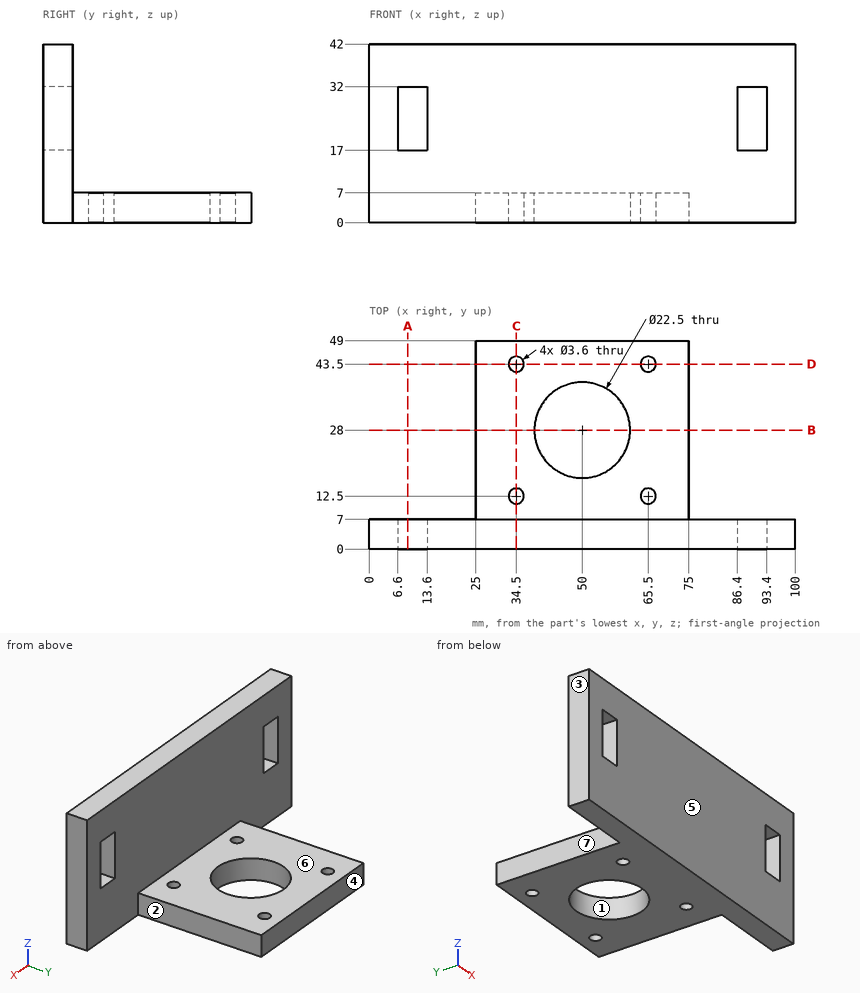
Job drawing, mm, ordinate dimensions from the low corner. One solid piece. A direction names the side the tool comes from. Give positions to 0.01 mm unless a question says otherwise; leave off trailing zeros. Order: outer loops, then holes, each group sorted by start corner. A loop starts at its lowest first (then second) coordinate and runs counter-clockwise, first axis right, second up. Notation, with made-up numbers: (15.5, 88.5) -> (38.5, 88.5) arc R23 ccw to (38.5, 99.5) -> close; hole circle Ø2 at (-12.5, -1). An arc over 180 degrees is marked (long way). Return JSON: item names as keys, results as strings.
Q1. Saw through at C-C (x = 34.5). Write the cut outline in (y, z), then the cut area to 3 significant figures.
Working result:
{"outline": "(0, 0) -> (10.7, 0) -> (10.7, 7) -> (7, 7) -> (7, 42) -> (0, 42) -> close; (14.3, 0) -> (41.7, 0) -> (41.7, 7) -> (14.3, 7) -> close; (45.3, 0) -> (49, 0) -> (49, 7) -> (45.3, 7) -> close", "area": "538 mm²"}
Q2. Mould opens along X. For the marked faces 1, 2, 3 and 4 say: pulls with the +X half, pulls with the -X half, needs draft (parallel to the pull), parting line crosses it, or undercut.
Working result:
{"face 1": "undercut", "face 2": "pulls with the +X half", "face 3": "pulls with the -X half", "face 4": "needs draft"}
Q3. Saw through at A-A (x = 9). Write the cut outline in (y, z), then the cut area to 3 significant figures.
Working result:
{"outline": "(0, 0) -> (7, 0) -> (7, 17) -> (0, 17) -> close; (0, 32) -> (7, 32) -> (7, 42) -> (0, 42) -> close", "area": "189 mm²"}
Q4. Flat gauge pins, fed straight in: pin 1 (12.5 mm diameter, centred on x = 41.5, y = 22, fed in from +Z); pin 2 (7.5 mm diameter, centred on y = 35.5, z = 2, fed in from +X); pin 3 (2 mm diameter, centred on y = 32, z = 4.5, fed in from -X). Where does each tip first touch, or does it go through?
Working result:
{"pin 1": "z = 7", "pin 2": "x = 75", "pin 3": "x = 25"}
Q5. Saw through at D-D (y = 43.5). Write the cut outline in (x, z), then the cut area to 3 significant figures.
Working result:
{"outline": "(25, 0) -> (32.7, 0) -> (32.7, 7) -> (25, 7) -> close; (36.3, 0) -> (63.7, 0) -> (63.7, 7) -> (36.3, 7) -> close; (67.3, 0) -> (75, 0) -> (75, 7) -> (67.3, 7) -> close", "area": "300 mm²"}
Q6. Saw through at B-B (y = 28). Write the cut outline in (x, z).
Working result:
{"outline": "(25, 0) -> (38.75, 0) -> (38.75, 7) -> (25, 7) -> close; (61.25, 0) -> (75, 0) -> (75, 7) -> (61.25, 7) -> close"}
Q7. Drill centre lines: line 1 (Y direction, x = 34.5, z = 2.5); line 2 (X direction, y = 4, z = 21); line 3 (X direction, y = 28.5, z = 6). Where is each one in solid material? Low to high.
Working result:
{"line 1": "0 to 10.7, 14.3 to 41.7, 45.3 to 49", "line 2": "0 to 6.6, 13.6 to 86.4, 93.4 to 100", "line 3": "25 to 38.76, 61.24 to 75"}
Q8. Which spindle directions (+Z, -Z, +X, -X, +Y, -Y) get a long thin tool onto all of the face, cutting with end or side? Do the marked faces 5, 6 and 7. Say none if no direction does.
Working result:
{"face 5": "+Z, -Z, +X, -X, -Y", "face 6": "+Z, +X, -X, +Y", "face 7": "+Z, -Z, -X, +Y"}
